from build123d import *

# Parameters (mm, degrees)
SKETCH1_W           = 13.97
SKETCH1_H           = 34.925
BOSS_EXTRUDE1_DEPTH = 4.7625
SKETCH2_W           = 6.35
SKETCH2_H           = 34.925
BOSS_EXTRUDE2_DEPTH = 14.2875
SKETCH3_R           = 1.4605
BOSS_EXTRUDE3_DEPTH = 11.5062
SKETCH4_R           = 1.9939
CUT_EXTRUDE1_DEPTH  = 11.5062


with BuildPart() as part:
    # Sketch1 → Boss-Extrude1 (new body)
    with BuildSketch(Plane.XY.offset(25.4)):
        with Locations((-180.974999938, 108.007553269)):
            Rectangle(SKETCH1_W, SKETCH1_H)
    extrude(amount=BOSS_EXTRUDE1_DEPTH)

    # Sketch2 → Boss-Extrude2 (add)
    with BuildSketch(Plane.XY.offset(30.1625)):
        with Locations((-184.784999938, 108.007553269)):
            Rectangle(SKETCH2_W, SKETCH2_H)
    extrude(amount=BOSS_EXTRUDE2_DEPTH)

    # Sketch3 → Boss-Extrude3 (add)
    with BuildSketch(Plane.XY.offset(44.45)):
        with Locations((-184.784999938, 120.541132469)):
            Circle(SKETCH3_R)
        with Locations((-184.784999938, 108.007553269)):
            Circle(SKETCH3_R)
        with Locations((-184.784999938, 95.473974069)):
            Circle(SKETCH3_R)
    extrude(amount=BOSS_EXTRUDE3_DEPTH)

    # Sketch4 → Cut-Extrude1 (cut)
    with BuildSketch(Plane.XY.offset(30.1625)):
        with Locations((-177.799999938, 95.244053269)):
            Circle(SKETCH4_R)
        with Locations((-177.799999938, 107.944053269)):
            Circle(SKETCH4_R)
        with Locations((-177.799999938, 120.644053269)):
            Circle(SKETCH4_R)
    extrude(amount=-CUT_EXTRUDE1_DEPTH, mode=Mode.SUBTRACT)


solid = part.part
Geometry: final body of the model. Coordinates: model frame, mm. A direction names the side the tool comes from. Coordinates: 2 decimals unless noted, no trailing zeros. Order: outer loops, then holes, each group sorted by start corner. A loop starts at its lowest first (then second) coordinate and runs counter-clockwise, first axis right, second up.
1) First-contact query: P1, Ø11.5, axis at y = 101.5, z = 36, coming from the +X side; P2, Ø2.5, axis at x = -177.8, y = 107.94, coming from the +Z side; P3, Ø5, axis at x = -184.5, z = 47, coming from the +Y side; P4, Ø6, axis at x = -177.5, y = 110, coming from the +Z side. Flat tips, straight axial feed; report the tip coordinate or a pass-through.
Result sheet:
P1: stops at x = -181.61
P2: passes through
P3: stops at y = 122
P4: stops at z = 30.16
2) Ray query, probe 1 along Y at (x, z) = (-177.8, 28.2); probe 2 along Y at (x, z) = (-178.75, 29); probe 3 along X at (y, z) = (108, 50.5). Return the intervals inside material, ascending.
Result sheet:
probe 1: y = 90.55 to 93.25, 97.24 to 105.95, 109.94 to 118.65, 122.64 to 125.47
probe 2: y = 90.55 to 93.49, 97 to 106.19, 109.7 to 118.89, 122.4 to 125.47
probe 3: x = -186.25 to -183.32
3) Section A-A (x = -177.8). Return loops of the section in (y, z), then the cut area to 3 significant figures.
Result sheet:
outline: (90.55, 25.4) - (93.25, 25.4) - (93.25, 30.16) - (90.55, 30.16) - close; (97.24, 25.4) - (105.95, 25.4) - (105.95, 30.16) - (97.24, 30.16) - close; (109.94, 25.4) - (118.65, 25.4) - (118.65, 30.16) - (109.94, 30.16) - close; (122.64, 25.4) - (125.47, 25.4) - (125.47, 30.16) - (122.64, 30.16) - close
area: 109 mm2
4) Set-up query: faces 1 (the flat face through (-185, 95, 55.956)), 2 (the flat face through (-181.61, 108, 37)), 3 (the cylindrical face through (-186.244, 120.605, 50.123)). Return all of +Z, -Z, +X, -X, +Y, -Y with unobstructed straight access to the full face (end or side cutting, diameter ignored); none if empty.
Result sheet:
face 1: +Z, +X, -X, +Y, -Y
face 2: +Z, +X, +Y, -Y
face 3: +Z
5) Section D-D (z = 48). Return loops of the section in (x, y) (1 decimal), then the cut area to 3 significant figures.
Result sheet:
outline: circle Ø2.9 at (-184.8, 95.5); circle Ø2.9 at (-184.8, 108); circle Ø2.9 at (-184.8, 120.5)
area: 20.1 mm2
6) Section C-C (y = 112.5). Return loops of the section in (x, z).
Result sheet:
outline: (-187.96, 25.4) - (-173.99, 25.4) - (-173.99, 30.16) - (-181.61, 30.16) - (-181.61, 44.45) - (-187.96, 44.45) - close
7) Section B-B (y = 120). Return loops of the section in (x, z).
Result sheet:
outline: (-187.96, 25.4) - (-179.69, 25.4) - (-179.69, 30.16) - (-181.61, 30.16) - (-181.61, 44.45) - (-183.43, 44.45) - (-183.43, 55.96) - (-186.14, 55.96) - (-186.14, 44.45) - (-187.96, 44.45) - close; (-175.91, 25.4) - (-173.99, 25.4) - (-173.99, 30.16) - (-175.91, 30.16) - close
8) Draft query along X for faces 4 (the cylindrical face through (-186.244, 108.072, 50.123)), 5 (the flat face through (-180, 108, 30.162)), 6 (the cylindrical face through (-175.96, 119.88, 27.81)). Return one class per face: released by +X, released by -X, zero draft, split by the parting line, or undercut.
Result sheet:
face 4: split by the parting line
face 5: zero draft
face 6: undercut
